Check sheet for the modelled part. Datum: model origin and axes. Units: mm. Face numbers are marked on the shaded views. A direction names the side the tool comes from. Round coordinates to 2 decimals unless told otherwise and drop trailing zeros. Write each loop counter-clockwise with the first axis right and the second up, starting at its lowest first coordinate (ties: lowest second). Pieces come first, ordered by that corner, then holes.
Item 1: Cross-section at D-D on z = 63. Enter the section's corners in (x, y).
Item 2: Tool access check on the marked faces 5 and 6. Record the directions out of +Z, -Z, +X, -X, +Y, -Y that give a thin tool (end or side, any length) a straight path to the whole face; none if there is none.
Item 3: Cross-section at A-A on x = 0. Enter the section's corners in (y, z).
Item 4: Go/stop test with flat-tipped pins: pin 1 Ø17 at (x, y) = (0, 50) entering from +Z; pin 2 Ø2 at (x, z) = (45, 61.5) entering from +Y. Record where each tip stops, or that it passes through.
Item 5: Material ranges on line 1 (X direction, y = 64, z = 62); line 2 (Y direction, x = 51, z = 50); line 3 (Z direction, x = 35.5, y = 9.5), recorded low to high.
Item 6: Cross-section at C-C on y = 50. Enter the section's corners in (x, z), plus the area to 3 significant figures.
Item 7: Cross-section at B-B on z = 50. Enter the section's corners in (x, y), plus the area to 3 significant figures.
Item 8: Release check for a two-part mould opening along X. For the marked faces 1, 2, 3 and 4 record: +X half, -X half, draft (parallel to the pull), parting line (faces both ways), or undercut.
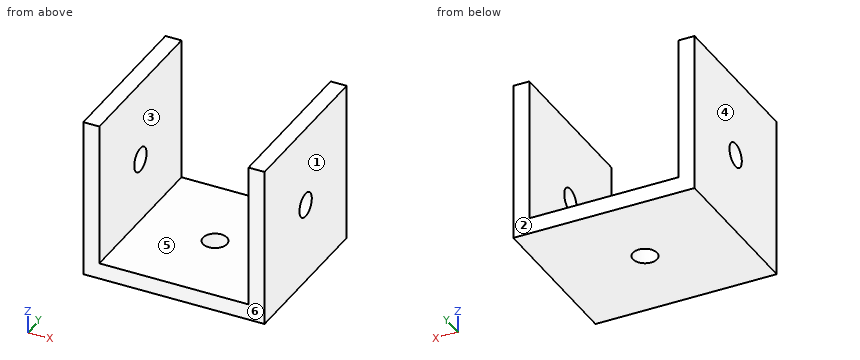
from build123d import *

# Parameters (mm, degrees)
BOSS_EXTRUDE1_DEPTH = 100
SKETCH2_R           = 7.5
CUT_EXTRUDE1_DEPTH  = 140
SKETCH3_R           = 7.5
CUT_EXTRUDE2_DEPTH  = 140


with BuildPart() as part:
    # Sketch1 → Boss-Extrude1 (new body)
    with BuildSketch(Plane(origin=(0, 0, 0), x_dir=(1, 0, 0), z_dir=(0, 1, 0))):
        Polygon((-56.5, 0), (56.5, 0), (56.5, -100), (46.5, -100), (46.5, -10), (-46.5, -10), (-46.5, -100), (-56.5, -100), align=None)
    extrude(amount=BOSS_EXTRUDE1_DEPTH)

    # Sketch2 → Cut-Extrude1 (cut)
    with BuildSketch(Plane(origin=(56.5, 0, 0), x_dir=(0, 0, -1), z_dir=(1, 0, 0))):
        with Locations((-50, 50)):
            Circle(SKETCH2_R)
    extrude(amount=-CUT_EXTRUDE1_DEPTH, mode=Mode.SUBTRACT)

    # Sketch3 → Cut-Extrude2 (cut)
    with BuildSketch(Plane(origin=(0, 0, 0), x_dir=(-1, 0, 0), z_dir=(0, 0, -1))):
        with Locations((0, 50)):
            Circle(SKETCH3_R)
    extrude(amount=-CUT_EXTRUDE2_DEPTH, mode=Mode.SUBTRACT)


solid = part.part
Response values:
1. outline: (-56.5, 0) - (-46.5, 0) - (-46.5, 100) - (-56.5, 100) - close; (46.5, 0) - (56.5, 0) - (56.5, 100) - (46.5, 100) - close
2. face 5: +Z, +Y, -Y
2. face 6: +Z, -Z, +X, -X, -Y
3. outline: (0, 0) - (42.5, 0) - (42.5, 10) - (0, 10) - close; (57.5, 0) - (100, 0) - (100, 10) - (57.5, 10) - close
4. pin 1: stops at z = 10
4. pin 2: passes through
5. line 1: x = -56.5 to -46.5, 46.5 to 56.5
5. line 2: y = 0 to 42.5, 57.5 to 100
5. line 3: z = 0 to 10
6. outline: (-56.5, 0) - (-7.5, 0) - (-7.5, 10) - (-46.5, 10) - (-46.5, 42.5) - (-56.5, 42.5) - close; (-56.5, 57.5) - (-46.5, 57.5) - (-46.5, 100) - (-56.5, 100) - close; (7.5, 0) - (56.5, 0) - (56.5, 42.5) - (46.5, 42.5) - (46.5, 10) - (7.5, 10) - close; (46.5, 57.5) - (56.5, 57.5) - (56.5, 100) - (46.5, 100) - close
6. area: 2,480 mm2
7. outline: (-56.5, 0) - (-46.5, 0) - (-46.5, 42.5) - (-56.5, 42.5) - close; (-56.5, 57.5) - (-46.5, 57.5) - (-46.5, 100) - (-56.5, 100) - close; (46.5, 0) - (56.5, 0) - (56.5, 42.5) - (46.5, 42.5) - close; (46.5, 57.5) - (56.5, 57.5) - (56.5, 100) - (46.5, 100) - close
7. area: 1,700 mm2
8. face 1: +X half
8. face 2: draft
8. face 3: undercut
8. face 4: -X half
